Build history of the part. All positions in model axes, mm. Coordinates: 2 decimals unless noted, no trailing zeros. Write each question's results on one line, items separated by ' | '. Start each with the question number.
Q1. Saw through at A-A on x = -2. Count the separate pieces of the cut face and the enclosed holes in it, and give its area (3 significant figures).
Q2. Two-plate mould, pull along Y, no slides. Class faces 1 (the face through (0.54, 2.44, 2.54)), 2 (the face through (0, 11, 5)), 3 (the face through (5.82, -4.79, 2.54)): released by +Y, released by -Y, zero draft, split by the parting line, or undercut.
Q3. Drill centre lines: line 1 (Y direction, x = 0, z = 1.3); line 2 (X direction, y = 1.5, z = 3.9). Where is each one in solid material? Low to high.
Q4. Drop flat-ended pins along their axis: pin 1 Ø3 at (y, z) = (-3.5, 4.5) entering from -X; pin 2 Ø4 at (x, y) = (0, 0) entering from +Z; pin 3 Ø1 at (y, z) = (12, 1) entering from +X; pin 4 Ø2 at (y, z) = (22, 1.5) entering from -X. Give the stop position or say it passes through.
from build123d import *

# Parameters (mm, degrees)
CROQUIS1_R              = 2.499999999
SALIENTE_EXTRUIR1_DEPTH = 5


with BuildPart() as part:
    # Croquis1 → Saliente-Extruir1 (new body)
    with BuildSketch(Plane.XY.offset(5)):
        with BuildLine():
            ThreePointArc((-1.502391268, 27.446296254), (-10.857150944, 26.658474231), (-5.165151301, 19.192998211))
            add(Edge.make_bspline(
                [(-5.165151301, 19.192998211), (0.561959139, 18.161248815), (-2.0209311, 9.093501776), (-7.220176541, 0.935588497), (-5.098734301, -5.629541665), (-2.791423521, -7.000958644)],
                knots=[0, 0, 0, 0, 0.419324493, 0.73408421, 1, 1, 1, 1], degree=3))
            ThreePointArc((-2.791423521, -7.000958644), (5.90367611, -4.685304218), (6.184039559, 4.308494165))
            add(Edge.make_bspline(
                [(6.184039559, 4.308494165), (3.613892894, 7.929527917), (3.595744884, 16.916271928), (0.755595428, 23.472120645), (-1.502391268, 27.446296254)],
                knots=[0, 0, 0, 0, 0.531518306, 1, 1, 1, 1], degree=3))
        make_face()
        with Locations(Location((1e-09, 1e-09, 0), (0, 0, 180))):
            Circle(CROQUIS1_R, mode=Mode.SUBTRACT)
    extrude(amount=-SALIENTE_EXTRUIR1_DEPTH)


solid = part.part
Returned:
1) separate pieces: 3 | enclosed holes: 0 | area: 127 mm2
2) face 1: undercut | face 2: zero draft | face 3: split by the parting line
3) line 1: y = -7.54 to -2.5, 2.5 to 24.66 | line 2: x = -5.79 to -2, 2 to 7.39
4) pin 1: stops at x = -5.84 | pin 2: passes through | pin 3: stops at x = 3.63 | pin 4: stops at x = -11.11
